Can you work these out from the model? Positions are in its coordinate system, mm. Face numbers are marked on the shaded views. Give positions to 0.01 mm unless a question says otherwise; leave off trailing zeros. Write each loop counter-clockwise with the first axis right and the second up, starting at its lowest first coordinate (ties: lowest second). Pieces come first, ordered by that corner, then holes.
1. I'm going to push a flat-ended pin straight in: pin 1 (3 mm diameter, centred on x = -13, y = -3.5, fed in from -Z). Where does the tip first touch, or does it pass through?
2. Suppose I cut it at C-C (z = 70). Please give me the cut outline in (x, y).
3. Thinking about a two-plate mould opening in Y: for the marked faces 1, 2 and 3, which applies, pulls with the +Y half, pulls with the -Y half, needs draft (parallel to the pull), parting line crosses it, or undercut?
4. Suppose I cut it at A-A (y = -21). Please give me the cut outline in (x, z).
5. If I drill on probe 1 along X at (y, z) = (-12.25, -11); probe 2 along X at (y, z) = (-23, -9); probe 3 along Z at (x, y) = (-55, -2.25), over which ranges is the centre line in solid material (lowest first)?
6. Suppose I cut it at B-B (y = -11.25). Please give me the cut outline in (x, z), and give its area (3 significant figures).
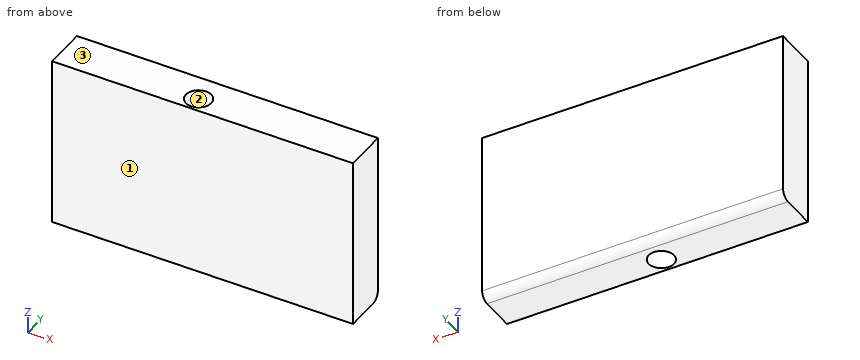
```python
from build123d import *

# Parameters (mm, degrees)
F0_W     = 177.8
F0_H     = 101.6
F1_DEPTH = 25.4
F2_R     = 7.5
F3_DEPTH = 150
F4_R     = 5


with BuildPart() as f1:
    # F0 (on Front) → F1 (new body)
    with BuildSketch(Plane.XZ):
        with Locations((-51.646665, 27.939998)):
            Rectangle(F0_W, F0_H)
    extrude(amount=F1_DEPTH)

    # F2 (on face) → F3 (cut)
    with BuildSketch(Plane.XY.offset(78.739998)):
        with Locations((-59.266985, -16.284161)):
            Circle(F2_R)
    extrude(amount=-F3_DEPTH, mode=Mode.SUBTRACT)

    # F4
    f4_edges = [f1.edges().sort_by_distance(p)[0] for p in [
        (-51.646665, 0, -22.860002),
    ]]
    fillet(f4_edges, radius=F4_R)


solid = f1.part
```
Checks:
1. pin 1: stops at z = -22.86
2. outline: (-140.55, -25.4) - (37.25, -25.4) - (37.25, 0) - (-140.55, 0) - close; hole circle Ø15 at (-59.27, -16.28)
3. face 1: pulls with the -Y half
3. face 2: undercut
3. face 3: needs draft
4. outline: (-140.55, -22.86) - (-65.1, -22.86) - (-65.1, 78.74) - (-140.55, 78.74) - close; (-53.44, -22.86) - (37.25, -22.86) - (37.25, 78.74) - (-53.44, 78.74) - close
5. probe 1: x = -140.55 to -65.59, -52.94 to 37.25
5. probe 2: x = -140.55 to -62.61, -55.93 to 37.25
5. probe 3: z = -22.04 to 78.74
6. outline: (-140.55, -22.86) - (-64.83, -22.86) - (-64.83, 78.74) - (-140.55, 78.74) - close; (-53.71, -22.86) - (37.25, -22.86) - (37.25, 78.74) - (-53.71, 78.74) - close
6. area: 16,900 mm2
